Check sheet for the modelled part. Datum: model origin and axes. Units: mm. A direction names the side the tool comes from. Give positions to 0.01 mm unless a question says otherwise; leave off trailing zeros. Loops run counter-clockwise (first coordinate to the right, second up) from the corner with the lowest first, then second, coordinate; pieces in that order, holes last. Notation, with made-up numbers: (47, -12.5) -> (80, -12.5) arc R19 ccw to (80, 4.5) -> close; hole circle Ø7 at (50.5, -5). An arc over 180 degrees is marked (long way). Write each question's results on one line, items separated by ' | '. Start each with the question number.
1. Mould release check, pull along X, two halves, no side actions. Record for faces 3 (the face through (0, -10, 15.5)), 4 (the face through (15.5, -10, 0)), 5 (the face through (0, -10, -30)), 6 (the face through (-22.099, -9.86, 19.816)): +X half, -X half, draft (parallel to the pull), parting line (faces both ways), or undercut.
2. Cross-section at C-C on x = 0. Record the boundary of the cut face in (y, z), and give its area (3 significant figures).
3. Gauge pin test, flat ends, axial feed: pin 1 Ø13 at (x, z) = (0, -22) entering from +Y; pin 2 Ø10 at (x, y) = (16.5, -17.5) entering from +Z; pin 3 Ø5 at (y, z) = (-11.5, -22) entering from -X; pin 4 Ø2 at (x, y) = (-4.5, -16) entering from +Z. Record the tip position at first contact, or that the pin passes through.
4. Cross-section at D-D on y = -10. Count the separate pieces of the cut face and the enclosed holes in it, and give its area (3 significant figures).
5. Material ranges on L1, parallel to Z at x = 0, y = -5; L2, parallel to Z at x = -3, y = -15.25; L3, parallel to X at y = -8.25, z = -6, recorded low to high. Write a range as from..to.
6. Cross-section at B-B on y = -15.5. Record the boundary of the cut face in (x, z).
7. Cross-section at A-A on z = -6. Record the boundary of the cut face in (x, y), and give its area (3 significant figures).
8. Tool access check on faces 1 (the face through (22.12, -9.86, 19.764)), 2 (the face through (-15.5, -5, 0)). Record the directions out of +Z, -Z, +X, -X, +Y, -Y that give a thin tool (end or side, any length) a straight path to the whole face; none if there is none.
from build123d import *

# Parameters (mm, degrees)
F0_R     = 30
F0_W     = 31
F0_H     = 31
F1_DEPTH = 20
F2_R     = 4
F3_DEPTH = 48.3
F4_W     = 47.4329847097
F4_H     = 80
F4_W_2   = 35.6862902641
F5_DEPTH = 29.8
F6_R     = 4.5
F7_DEPTH = 22.501
F8_R     = 2
F9_DEPTH = 20.001
F10_R    = 5
F11_R    = 5


with BuildPart() as f1:
    # F0 (on Front) → F1 (new body)
    with BuildSketch(Plane.XZ):
        Circle(F0_R)
        Rectangle(F0_W, F0_H, mode=Mode.SUBTRACT)
    extrude(amount=F1_DEPTH)

    # F2 (on Front) → F3 (cut)
    with BuildSketch(Plane.XZ):
        with Locations((0, 22)):
            Circle(F2_R)
        with Locations((0, -22)):
            Circle(F2_R)
    extrude(amount=F3_DEPTH, mode=Mode.SUBTRACT)

    # F4 (on Front) → F5 (cut)
    with BuildSketch(Plane.XZ):
        with Locations((-46.2164923549, 0)):
            Rectangle(F4_W, F4_H)
        with Locations((40.3431451321, 0)):
            Rectangle(F4_W_2, F4_H)
    extrude(amount=F5_DEPTH, mode=Mode.SUBTRACT)

    # F6 (on Right) → F7 (cut, through all)
    with BuildSketch(Plane.YZ):
        with Locations((-10, 0)):
            Circle(F6_R)
    extrude(amount=-F7_DEPTH, mode=Mode.SUBTRACT)

    # F8 (on Front) → F9 (cut, through all)
    with BuildSketch(Plane.XZ):
        with Locations((-14.2, 14.2)):
            Circle(F8_R)
        with Locations((14.2, 14.2)):
            Circle(F8_R)
        with Locations((-14.2, -14.2)):
            Circle(F8_R)
        with Locations((14.2, -14.2)):
            Circle(F8_R)
    extrude(amount=F9_DEPTH, mode=Mode.SUBTRACT)

    # F10
    f10_edges = [f1.edges().sort_by_distance(p)[0] for p in [
        (-12.680132, -10, 15.5),
        (-15.5, -10, 12.680132),
        (12.680132, -10, 15.5),
        (15.5, -10, 12.680132),
        (15.5, -10, -12.680132),
        (12.680132, -10, -15.5),
        (-12.680132, -10, -15.5),
        (-15.5, -10, -12.680132),
    ]]
    fillet(f10_edges, radius=F10_R)

    # F11
    f11_edges = [f1.edges().sort_by_distance(p)[0] for p in [
        (-22.5, -10, 19.843135),
        (-22.5, -10, -19.843135),
        (22.5, -10, 19.843135),
        (22.5, -10, -19.843135),
    ]]
    fillet(f11_edges, radius=F11_R)


solid = f1.part
Geometry says:
1) face 3: undercut | face 4: undercut | face 5: parting line | face 6: -X half
2) outline: (-20, -30) -> (0, -30) -> (0, -26) -> (-20, -26) -> close; (-20, -18) -> (0, -18) -> (0, -15.5) -> (-20, -15.5) -> close; (-20, 15.5) -> (0, 15.5) -> (0, 18) -> (-20, 18) -> close; (-20, 26) -> (0, 26) -> (0, 30) -> (-20, 30) -> close | area: 260 mm^2
3) pin 1: y = 0 | pin 2: z = 27.71 | pin 3: x = -22.22 | pin 4: z = 29.8
4) separate pieces: 1 | enclosed holes: 2 | area: 1,280 mm^2
5) L1: -30..-26, -18..-15.5, 15.5..18, 26..30 | L2: -29.85..-24.65, -19.35..-15.5, 15.5..19.35, 24.65..29.85 | L3: -22.5..-15.5, 15.5..22.5
6) outline: (-22.5, -17.85) arc R5 ccw to (-21, -21.42) arc R30 ccw to (21, -21.42) arc R5 ccw to (22.5, -17.85) -> (22.5, 17.85) arc R5 ccw to (21, 21.42) arc R30 ccw to (-21, 21.42) arc R5 ccw to (-22.5, 17.85) -> close; hole (-16, -13.33) arc R2 ccw to (-13.33, -16) arc R5 cw to (-11.15, -15.5) -> (11.15, -15.5) arc R5 cw to (13.33, -16) arc R2 ccw to (16, -13.33) arc R5 cw to (15.5, -11.15) -> (15.5, 11.15) arc R5 cw to (16, 13.33) arc R2 ccw to (13.33, 16) arc R5 cw to (11.15, 15.5) -> (-11.15, 15.5) arc R5 cw to (-13.33, 16) arc R2 ccw to (-16, 13.33) arc R5 cw to (-15.5, 11.15) -> (-15.5, -11.15) arc R5 cw to start; hole circle Ø8 at (0, -22); hole circle Ø8 at (0, 22)
7) outline: (-22.5, -20) -> (-15.5, -20) -> (-15.5, 0) -> (-22.5, 0) -> close; (15.5, -20) -> (22.5, -20) -> (22.5, 0) -> (15.5, 0) -> close | area: 280 mm^2
8) face 1: +Z, +X, +Y, -Y | face 2: +Y, -Y
